```python
from build123d import *

# Parameters (mm, degrees)
EXTRUDE_2_DEPTH     = 26.8
SHELL_2_T           = 3
F_3_0MM_1_D         = 3
F_3_0MM_1_DEPTH     = 5
F_3_0MM_1_TIP       = 0.901290929
F_3_0MM_2_D         = 5.5
F_3_0MM_2_DEPTH     = 1.5
F_3_0MM_2_TIP       = 1.652366702
SKETCH_16_W         = 5
SKETCH_16_H         = 2.7
CUT_EXTRUDE_3_DEPTH = 10


with BuildPart() as part:
    # 草图2 → 凸台-拉伸2 (new body)
    with BuildSketch(Plane(origin=(0, 0, 0), x_dir=(1, 0, 0), z_dir=(0, 1, 0))):
        Polygon((0, 0), (46, 0), (46, 23), (26.000191801, 42.999808199), (26.000191801, 48.999808199), (46, 68.999616398), (46, 91.999616398), (0, 91.999616398), (0, 68.999616398), (19.999808199, 48.999808199), (19.999808199, 42.999808199), (0, 23), align=None)
    extrude(amount=EXTRUDE_2_DEPTH)

    # 抽壳2
    shell_2_openings = [part.faces().sort_by_distance(p)[0] for p in [
        (23, 26.8, -45.999808199),
    ]]
    offset(amount=SHELL_2_T, openings=shell_2_openings, kind=Kind.INTERSECTION)

    # Ø3.0mm 暗销孔1
    with Locations(Plane(origin=(5, -3, -5), x_dir=(0, 0, -1), z_dir=(0, -1, 0))):
        with Locations((0, 0), (0, 36), (82, 36), (82, 0)):
            Hole(F_3_0MM_1_D / 2, depth=F_3_0MM_1_DEPTH)
            with Locations((0, 0, -(F_3_0MM_1_DEPTH + F_3_0MM_1_TIP / 2))):  # 118° drill point
                Cone(0, F_3_0MM_1_D / 2, F_3_0MM_1_TIP, mode=Mode.SUBTRACT)

    # Ø3.0mm 暗销孔2
    with Locations(Plane(origin=(5, -3, -5), x_dir=(0, 0, -1), z_dir=(0, -1, 0))):
        with Locations((0, 0), (0, 36), (82, 36), (82, 0)):
            Hole(F_3_0MM_2_D / 2, depth=F_3_0MM_2_DEPTH)
            with Locations((0, 0, -(F_3_0MM_2_DEPTH + F_3_0MM_2_TIP / 2))):  # 118° drill point
                Cone(0, F_3_0MM_2_D / 2, F_3_0MM_2_TIP, mode=Mode.SUBTRACT)

    # 草图16 → 切除-拉伸3 (cut)
    with BuildSketch(Plane(origin=(0, 0, 0), x_dir=(0, 0, -1), z_dir=(1, 0, 0))):
        with Locations((15, 12.95)):
            Rectangle(SKETCH_16_W, SKETCH_16_H)
    extrude(amount=-CUT_EXTRUDE_3_DEPTH, mode=Mode.SUBTRACT)


solid = part.part
```
For this review, take the finished solid that the model builds, in its own axes (mm). A direction names the side the tool comes from. Give positions to 0.01 mm unless a question says otherwise; leave off trailing zeros. Loops run counter-clockwise (first coordinate to the right, second up) from the corner with the lowest first, then second, coordinate; pieces in that order, holes last. Notation, with made-up numbers: M 76.5,27 L 135.5,27 A7 ccw 135.5,32 Z; hole C 31.5,22 d2. An arc over 180 degrees is marked long. One line per item, written item: value. Start each with the question number.
Q1. Add section B-B (x = 41). Count the separate pieces of the cut face and the enclosed holes in it, and give its area (3 significant figures).
Q2. Clearance check with flat-ended pins moving along their axes: pin 1 Ø6.5 at (x, z) = (5, -5) entering from +Y; pin 2 Ø3.5 at (x, z) = (41, -87) entering from -Y; pin 3 Ø1.8 at (y, z) = (9, -45.5) entering from +X. State where each tip first meets the part, or that it passes through.
Q3. Add section C-C (y = 10.5). Give the boundary of the cut face in (x, z), and give its area (3 significant figures).
Q4. Add section D-D (x = 23.5). Give the boundary of the cut face in (y, z), and give its area (3 significant figures).
Q5. Machinability: for faces 4 (the face through (29, 12, -46)), 5 (the face through (23, 13, -92)), 6 (the face through (6.86, 11.691, -57.897)), 7 (the face through (-1, 13, -12.5)), which of the approach directions +Z, -Z, +X, -X, +Y, -Y give a long, thin tool a straight path to every point of the face, cutting with its end or side? Answer none if there is none.
Q6. Draft analysis for pull direction Y (two halves, no side actions). For faces 1 (the face through (39.67, -0.37, -86.31)), 2 (the face through (23, 0, -47)), 3 (the face through (-1, 11.6, -15)), state which applies: released by +Y, released by -Y, zero draft, split by the parting line, or undercut.
Q7. For L1, parallel to X at y = -2.3, z = -87; L2, parallel to X at y = -0.3, z = -87; L3, parallel to X at y = 22.75, z = -3, list the stretches that pass through material, from the lowest coordinate up.
Q8. Add section A-A (z = -5). Give the boundary of the cut face in (x, y), and give its area (3 significant figures).
Reply:
1. separate pieces: 4
1. enclosed holes: 0
1. area: 572 mm²
2. pin 1: y = 0
2. pin 2: y = -0.9
2. pin 3: x = 29
3. outline: M -3,-95 L 49,-95 L 49,-67.76 L 29,-47.76 L 29,-44.24 L 49,-24.24 L 49,3 L -3,3 L -3,-24.24 L 17,-44.24 L 17,-47.76 L -3,-67.76 Z; hole M 0,-92 L 46,-92 L 46,-69 L 26,-49 L 26,-43 L 46,-23 L 46,0 L 0,0 L 0,-23 L 20,-43 L 20,-49 L 0,-69 Z
3. area: 963 mm²
4. outline: M -3,-95 L 26.8,-95 L 26.8,-92 L 0,-92 L 0,0 L 26.8,0 L 26.8,3 L -3,3 Z
4. area: 455 mm²
5. face 4: +X, +Y, -Y
5. face 5: +Y
5. face 6: -X, +Y, -Y
5. face 7: -X
6. face 1: zero draft
6. face 2: released by +Y
6. face 3: undercut
7. L1: -3 to 2.25, 7.75 to 38.25, 43.75 to 49
7. L2: -3 to 3.5, 6.5 to 39.5, 42.5 to 49
7. L3: -3 to 0, 46 to 49
8. outline: M -3,-3 L 2.25,-3 L 2.25,-1.5 L 3.5,-0.75 L 3.5,0 L 0,0 L 0,26.8 L -3,26.8 Z; M 6.5,-0.75 L 7.75,-1.5 L 7.75,-3 L 38.25,-3 L 38.25,-1.5 L 39.5,-0.75 L 39.5,0 L 6.5,0 Z; M 42.5,-0.75 L 43.75,-1.5 L 43.75,-3 L 49,-3 L 49,26.8 L 46,26.8 L 46,0 L 42.5,0 Z
8. area: 289 mm²
